Source: CAD feature listing. Evaluate the final solid. Frame: model axes, mm. A direction names the side the tool comes from. Coordinates: 2 decimals unless noted, no trailing zeros. Order: outer loops, then holes, each group sorted by start corner. A loop starts at its lowest first (then second) coordinate and runs counter-clockwise, first axis right, second up. Notation, with made-up numbers: (18, 24.25) -> (63, 24.25) arc R5 cw to (63, 31.25) -> close; hole circle Ø8 at (84.5, -39). An arc over 180 degrees is marked (long way). Put each result on its own line as item: value.
Autodesk Inventor part; units mm, degrees
ref_plane "YZ Plane" through (0, 0, 0) normal (1, 0, 0) x (0, 1, 0)
ref_plane "XZ Plane" through (0, 0, 0) normal (0, 1, 0) x (-1, 0, 0)
ref_plane "XY Plane" through (0, 0, 0) normal (0, 0, 1) x (1, 0, 0)
sketch "Sketch1" plane through (0, 0, 0) normal (1, 0, 0) x (0, 1, 0)
  circle A0 centre (0, 0) radius 2
  line L0 (-20.007, 88.601) -> (-20.007, 57.351)
  line L1 (-20.007, 57.351) -> (-25.007, 57.351)
  line L2 (-25.007, 88.601) -> (-25.007, 57.351)
  line L3 (-20.007, 88.601) -> (-25.007, 88.601)
  line L4 (-20.007, 31.101) -> (-20.007, -31.899)
  line L5 (-20.007, -31.899) -> (-25.007, -31.899)
  line L6 (-25.007, 31.101) -> (-25.007, -31.899)
  line L7 (-20.007, 31.101) -> (-25.007, 31.101)
  line L8 (-20.007, -58.149) -> (-20.007, -89.399)
  line L9 (-20.007, -89.399) -> (-25.007, -89.399)
  line L10 (-25.007, -58.149) -> (-25.007, -89.399)
  line L11 (-20.007, -58.149) -> (-25.007, -58.149)
  line L12 (19.993, 93.601) -> (19.993, 98.601)
  line L13 (19.993, 98.601) -> (9.9915, 98.601)
  line L14 (9.9915, 93.601) -> (9.9915, 98.601)
  line L15 (-10.0085, 93.601) -> (-10.0085, 98.601)
  line L16 (-25.0077, 98.601) -> (-10.0085, 98.601)
  line L17 (-25.007, 93.601) -> (-25.007, 98.601)
  line L18 (-25.007, 93.601) -> (-33.007, 93.601)
  line L19 (-33.007, 93.601) -> (-33.007, -94.399)
  line L20 (-10.0085, 93.601) -> (9.9915, 93.601)
  line L21 (24.993, -99.399) -> (24.993, -94.399)
  line L22 (9.993, -99.399) -> (24.993, -99.399)
  line L23 (9.993, -99.399) -> (9.993, -94.399)
  line L24 (-10.0077, -94.399) -> (9.993, -94.399)
  line L25 (-10.0077, -99.399) -> (-10.0077, -94.399)
  line L26 (-25.0077, -99.399) -> (-10.0077, -99.399)
  line L27 (-25.0077, -99.399) -> (-25.0077, -94.399)
  line L28 (-33.0079, -94.399) -> (-25.0077, -94.399)
  line L29 (19.993, 93.601) -> (24.993, 93.601)
  line L30 (24.993, -94.399) -> (24.993, -89.399)
  line L31 (21.993, -89.399) -> (24.993, -89.399)
  line L32 (21.993, -89.399) -> (21.993, -58.149)
  line L33 (21.993, -58.149) -> (24.993, -58.149)
  line L34 (24.993, -58.149) -> (24.993, -31.899)
  line L35 (21.993, -31.899) -> (24.993, -31.899)
  line L36 (21.993, -31.899) -> (21.993, 31.101)
  line L37 (21.993, 31.101) -> (24.993, 31.101)
  line L38 (24.993, 31.101) -> (24.993, 57.351)
  line L39 (21.993, 57.351) -> (24.993, 57.351)
  line L40 (21.993, 57.351) -> (21.993, 88.601)
  line L41 (21.993, 88.601) -> (24.993, 88.601)
  line L42 (24.993, 88.601) -> (24.993, 93.601)
  point P0 (-29.9123, 87.1698)
  dimension "d24" = 4
  dimension "d25" = 8
  dimension "d27" = 198
  dimension "d30" = 5
  dimension "d31" = 188
  dimension "d32" = 188
  dimension "d33" = 58
  dimension "d35" = 3
extrude "Extrusion1" add sketch "Sketch1" along normal blind 5
properties part number "case top sides" material "ABS Plastic"
1. Cut plane C-C on z = 0. Output: boundary loops of the cut face in (x, y).
Numbers:
outline: (0, -33.01) -> (5, -33.01) -> (5, -25.01) -> (0, -25.01) -> close; (0, -20.01) -> (5, -20.01) -> (5, -2) -> (0, -2) -> close; (0, 2) -> (5, 2) -> (5, 21.99) -> (0, 21.99) -> close
2. Cut plane A-A on y = 0. Output: boundary loops of the cut face in (x, z), plus the area to 3 significant figures.
Numbers:
outline: (0, -94.4) -> (5, -94.4) -> (5, -2) -> (0, -2) -> close; (0, 2) -> (5, 2) -> (5, 93.6) -> (0, 93.6) -> close
area: 920 mm2
3. Set-up query: faces 4 (the flat face through (2, -29, 93.601)), 5 (the flat face through (2, 0, 93.601)), 6 (the flat face through (2, -22, -58.149)), 7 (the flat face through (2, 21.993, -74)), 8 (the flat face through (2, -10.008, -97)). Return all of +Z, -Z, +X, -X, +Y, -Y with unobstructed straight access to the full face (end or side cutting, diameter ignored); none if empty.
Numbers:
face 4: +Z, +X, -X, -Y
face 5: +Z, +X, -X
face 6: +X, -X
face 7: +X, -X, +Y
face 8: -Z, +X, -X
4. Cut plane D-D on x = 1.2. Count the separate pieces of the cut face and the enclosed holes in it, plus the area to 3 significant figures.
Numbers:
separate pieces: 1
enclosed holes: 4
area: 10,200 mm2
5. Ray query, line 1 along Y through (x, z) = (1.35, 65.5); line 2 along Z through (x, y) = (2.6, 0); line 3 along Z through (x, y) = (3.6, 2.5). Return the intervals inside material, ascending.
Numbers:
line 1: y = -33.01 to -25.01, -20.01 to 21.99
line 2: z = -94.4 to -2, 2 to 93.6
line 3: z = -94.4 to 93.6
6. Cut plane B-B on z = 63. Output: boundary loops of the cut face in (x, y), plus the area to 3 significant figures.
Numbers:
outline: (0, -33.01) -> (5, -33.01) -> (5, -25.01) -> (0, -25.01) -> close; (0, -20.01) -> (5, -20.01) -> (5, 21.99) -> (0, 21.99) -> close
area: 250 mm2
7. Pull-direction query (Y, two-part tool) for faces 1 (the flat face through (2, -25.008, -97)), 2 (the flat face through (5, -4, 1)), 3 (the cylindrical face through (2, 0, 2)); classes: pulls with the +Y half, pulls with the -Y half, needs draft (parallel to the pull), parting line crosses it, or undercut.
Numbers:
face 1: pulls with the -Y half
face 2: needs draft
face 3: undercut
8. First-contact query: pin 1 (2.5 mm diameter, centred on y = 0, z = 0, fed in from -X); pin 2 (1.5 mm diameter, centred on x = 2.5, z = -76, fed in from +Y); pin 3 (2.5 mm diameter, centred on x = 3.5, z = 97.5, fed in from -Y). Flat tips, straight axial feed; report the tip coordinate or a pass-through.
Numbers:
pin 1: passes through
pin 2: stops at y = 21.99
pin 3: stops at y = -25.01
